Can you work these out from the model? Positions are in its coordinate system, mm. A direction names the side the tool comes from. Coordinates: 2 decimals unless noted, no trailing zeros. Loops run counter-clockwise (first coordinate to the right, second up) from the corner with the lowest first, then second, coordinate; pieces in that order, holes last.
```python
from build123d import *

# Parameters (mm, degrees)
F1_DEPTH = 2.54
F2_DEPTH = 0.127


# Not quite as in the source:
# - a feature names something its author has since deleted; it is built from what else it names


with BuildPart() as f1:
    # F0 (on Front) → F1 (new body, symmetric)
    with BuildSketch(Plane.XZ):
        with BuildLine():
            Line((14.1115041016, 7.2841788642), (17.5840938227, 7.2841788642))
            Line((17.5840938227, 7.2841788642), (12.6545671137, 27.1918801591))
            Line((12.6545671137, 27.1918801591), (12.6545671137, 16.3482450677))
            ThreePointArc((12.6545671137, 16.3482450677), (15.261577361, 14.4943512953), (16.2604214978, 11.4553160965))
            ThreePointArc((16.2604214978, 11.4553160965), (15.6916123075, 9.109243219), (14.1115041016, 7.2841788642))
        make_face()
        with BuildLine():
            Line((-4.5987749709, 27.1918801591), (-10.4762865467, 7.2841788642))
            Line((-10.4762865467, 7.2841788642), (-7.0264551949, 7.2841788642))
            ThreePointArc((-7.0264551949, 7.2841788642), (-7.1794052372, 12.0962388338), (-4.5987749709, 16.1606775766))
            Line((-4.5987749709, 16.1606775766), (-4.5987749709, 27.1918801591))
        make_face()
        with BuildLine():
            ThreePointArc((-4.5987749709, 16.1606775766), (-7.1794052372, 12.0962388338), (-7.0264551949, 7.2841788642))
            Line((-7.0264551949, 7.2841788642), (8.1640722191, 7.2841788642))
            ThreePointArc((8.1640722191, 7.2841788642), (6.5839640132, 9.109243219), (6.0151548229, 11.4553160965))
            Line((6.0151548229, 11.4553160965), (0.7099450795, 11.4553160965))
            Line((0.7099450795, 11.4553160965), (-4.5987749709, 11.4553160965))
            Line((-4.5987749709, 11.4553160965), (-4.5987749709, 16.1606775766))
        make_face()
        with BuildLine():
            Line((-10.4762865467, 7.2841788642), (-10.4762865467, 0))
            Line((-10.4762865467, 0), (17.5840938227, 0))
            Line((17.5840938227, 0), (17.5840938227, 7.2841788642))
            Line((17.5840938227, 7.2841788642), (14.1115041016, 7.2841788642))
            ThreePointArc((14.1115041016, 7.2841788642), (11.2751644394, 6.3345251354), (8.3919880677, 7.1307404918))
            ThreePointArc((8.3919880677, 7.1307404918), (0.6285539733, 1.7598537536), (-7.0264551949, 7.2841788642))
            Line((-7.0264551949, 7.2841788642), (-10.4762865467, 7.2841788642))
        make_face()
        with BuildLine():
            Line((-10.4762865467, 7.2841788642), (-10.4762865467, 0))
            Line((-10.4762865467, 0), (17.5840938227, 0))
            Line((17.5840938227, 0), (17.5840938227, 7.2841788642))
            Line((17.5840938227, 7.2841788642), (14.1115041016, 7.2841788642))
            ThreePointArc((14.1115041016, 7.2841788642), (11.2751644394, 6.3345251354), (8.3919880677, 7.1307404918))
            ThreePointArc((8.3919880677, 7.1307404918), (0.6285539733, 1.7598537536), (-7.0264551949, 7.2841788642))
            Line((-7.0264551949, 7.2841788642), (-10.4762865467, 7.2841788642))
        make_face()
    extrude(amount=F1_DEPTH, both=True)

    # F0 (on Front) → F2 (join, symmetric)
    with BuildSketch(Plane.XZ):
        with BuildLine():
            ThreePointArc((7.2737737734, 14.8184641943), (1.628753339, 18.0658576504), (-4.5987749709, 16.1606775766))
            Line((-4.5987749709, 16.1606775766), (-4.5987749709, 11.4553160965))
            Line((-4.5987749709, 11.4553160965), (0.7099450795, 11.4553160965))
            Line((0.7099450795, 11.4553160965), (6.0151548229, 11.4553160965))
            ThreePointArc((6.0151548229, 11.4553160965), (6.3401167864, 13.250788652), (7.2737737734, 14.8184641943))
        make_face()
        with BuildLine():
            ThreePointArc((7.2737737734, 14.8184641943), (6.3401167864, 13.250788652), (6.0151548229, 11.4553160965))
            Line((6.0151548229, 11.4553160965), (8.7471650108, 11.4553160965))
            ThreePointArc((8.7471650108, 11.4553160965), (8.2016302385, 13.220637488), (7.2737737734, 14.8184641943))
        make_face()
        with BuildLine():
            ThreePointArc((6.0151548229, 11.4553160965), (6.5839640132, 9.109243219), (8.1640722191, 7.2841788642))
            Line((8.1640722191, 7.2841788642), (8.4463453539, 7.2841788642))
            ThreePointArc((8.4463453539, 7.2841788642), (8.7776037503, 8.5930277501), (8.8890353081, 9.9385390058))
            ThreePointArc((8.8890353081, 9.9385390058), (8.8534904982, 10.7002377527), (8.7471650108, 11.4553160965))
            Line((8.7471650108, 11.4553160965), (6.0151548229, 11.4553160965))
        make_face()
        with BuildLine():
            Line((8.4463453539, 7.2841788642), (14.1115041016, 7.2841788642))
            ThreePointArc((14.1115041016, 7.2841788642), (15.6916123075, 9.109243219), (16.2604214978, 11.4553160965))
            ThreePointArc((16.2604214978, 11.4553160965), (15.261577361, 14.4943512953), (12.6545671137, 16.3482450677))
            ThreePointArc((12.6545671137, 16.3482450677), (9.7369184571, 16.3826821662), (7.2737737734, 14.8184641943))
            ThreePointArc((7.2737737734, 14.8184641943), (8.2016302385, 13.220637488), (8.7471650108, 11.4553160965))
            ThreePointArc((8.7471650108, 11.4553160965), (8.8534904982, 10.7002377527), (8.8890353081, 9.9385390058))
            ThreePointArc((8.8890353081, 9.9385390058), (8.7776037503, 8.5930277501), (8.4463453539, 7.2841788642))
        make_face()
    extrude(amount=F2_DEPTH, both=True)


solid = f1.part
```
(1) I want a section at C-C on y = -1.05. Write out the boundary of the cut face in (x, z), then the cut area to 3 significant figures.
Check values:
outline: (-10.48, 0) - (17.58, 0) - (17.58, 7.28) - (12.65, 27.19) - (12.65, 16.35) arc R5.12 cw (long way) to (8.39, 7.13) arc R8.18 cw to (-7.03, 7.28) - (8.16, 7.28) arc R5.12 cw to (6.02, 11.46) - (-4.6, 11.46) - (-4.6, 27.19) - (-10.48, 7.28) - close
area: 267 mm2
(2) If we mould it in two halves opening along X, with no side actions, what happens to faces 1 (the flat face through (-4.599, 0, 19)), 2 (the flat face through (17.584, 0, 4)), 3 (the flat face through (3, 2.54, 8)), 4 (the flat face through (-10.476, 0, 4))? For each: released by +X, released by -X, zero draft, split by the parting line, or undercut.
Check values:
face 1: undercut
face 2: released by +X
face 3: zero draft
face 4: released by -X
(3) I want a section at A-A on x = 12. Write out the boundary of the cut face in (y, z).
Check values:
outline: (-2.54, 0) - (2.54, 0) - (2.54, 6.41) - (-2.54, 6.41) - close; (-0.13, 7.28) - (0.13, 7.28) - (0.13, 16.5) - (-0.13, 16.5) - close
(4) I want a section at B-B on z = 5.75. Write out the boundary of the cut face in (x, y).
Check values:
outline: (-10.48, -2.54) - (-6.32, -2.54) - (-6.32, 2.54) - (-10.48, 2.54) - close; (7.74, -2.54) - (17.58, -2.54) - (17.58, 2.54) - (7.74, 2.54) - close
(5) I'm going to push flat-ended pins straight in: pin 1 (1.9 mm diameter, centred on x = 1, y = 1.5, fed in from +Z); pin 2 (2.5 mm diameter, centred on y = 0.5, z = 21, fed in from +X); pin 3 (2.5 mm diameter, centred on x = 0.5, y = -1, fed in from +Z). Where does each tip first touch, or does it pass through?
Check values:
pin 1: stops at z = 11.46
pin 2: stops at x = 14.5
pin 3: stops at z = 18.12
(6) I want a section at D-D on z = 14.25. Write out the boundary of the cut face in (x, y), then the cut area to 3 significant figures.
Check values:
outline: (-8.42, -2.54) - (-4.6, -2.54) - (-4.6, -0.13) - (15.43, -0.13) - (15.43, -2.54) - (15.86, -2.54) - (15.86, 2.54) - (15.43, 2.54) - (15.43, 0.13) - (-4.6, 0.13) - (-4.6, 2.54) - (-8.42, 2.54) - close
area: 26.7 mm2
(7) If I drill on probe 1 along X at (y, z) = (1.1, 9.25); probe 2 along X at (y, z) = (0.8, 17.75); probe 3 along Y at (x, z) = (1.5, 13), over which ranges is the centre line in solid material (lowest first)?
Check values:
probe 1: x = -9.9 to 6.51, 15.76 to 17.1
probe 2: x = -7.39 to -4.6, 12.65 to 14.99
probe 3: y = -0.13 to 0.13
(8) Which directions (+Z, -Z, +X, -X, +Y, -Y) give clear straight access to the entire face, cutting with the end or side of a thin tool? Please do faces 5 (the flat face through (12.655, 0, 22)), 6 (the flat face through (1, -1, 11.455)), 7 (the cylindrical face through (6.6, 1.32, 9.08)), 8 (the flat face through (3, 0, 0)).
Check values:
face 5: +Z, +Y, -Y
face 6: +Z, -Y
face 7: +Z, +Y
face 8: -Z, +X, -X, +Y, -Y
